from build123d import *

# Parameters (mm, degrees)
CYLINDER004_R     = 28
CYLINDER004_DEPTH = 10


with BuildPart() as cylinder004:
    # Cylinder004 → Cylinder004 (new body)
    with BuildSketch(Plane.XY.offset(86)):
        Circle(CYLINDER004_R)
    extrude(amount=CYLINDER004_DEPTH)


with BuildPart() as cut004:
    # Cone004 → Cone004 (revolve)
    with BuildSketch(Plane(origin=(0, 0, 87), x_dir=(1, 0, 0), z_dir=(0, -1, 0))):
        Polygon((0, 0), (32.6, 0), (33, 5), (0, 5), align=None)
    revolve(axis=Axis((0, 0, 87), (0, 0, 1)))

    # Cut004: cut Cylinder004
    add(cylinder004.part, mode=Mode.SUBTRACT)


solid = cut004.part
Read the model definition and answer for the solid it produces. Units are mm, in the model's axes. Coordinates: 2 decimals unless noted, no trailing zeros. Order: outer loops, then holes, each group sorted by start corner. A loop starts at its lowest first (then second) coordinate and runs counter-clockwise, first axis right, second up. Notation, with made-up numbers: (63.5, -6) -> (100.5, -6) arc R15 cw to (100.5, 23) -> close; hole circle Ø5 at (-2.5, 9.25). An arc over 180 degrees is marked (long way). Answer as a JSON object with one key per item and string values.
1) Each of these flat-tipped pins is pushed along its axis until it touches: pin 1 (12 mm diameter, centred on x = 3.5, y = -18, fed in from +Z); pin 2 (2 mm diameter, centred on y = -14.5, z = 89, fed in from -X). Where does it stop, or does it pass through?
Model answer:
{"pin 1": "passes through", "pin 2": "stops at x = -29.86"}
2) A cutting plane is placed at A-A, the plane y = 0. Determine the outline of the cut face in (x, z), plus the area to 3 significant figures.
Model answer:
{"outline": "(-33, 92) -> (-32.6, 87) -> (-28, 87) -> (-28, 92) -> close; (28, 87) -> (32.6, 87) -> (33, 92) -> (28, 92) -> close", "area": "48.0 mm²"}
3) A cutting plane is placed at C-C, the plane z = 90.6. Determine the outline of the cut face in (x, y).
Model answer:
{"outline": "circle Ø65.78 at (0, 0); hole circle Ø56 at (0, 0)"}
4) The mould has two halves that part along X. Classify faces 1 (the face through (-14.3, 24.3, 87)), 2 (the face through (25.865, -10.724, 89.465)), 3 (the face through (-7.07, -31.85, 87.31)): released by +X, released by -X, zero draft, split by the parting line, or undercut.
Model answer:
{"face 1": "zero draft", "face 2": "undercut", "face 3": "split by the parting line"}
5) Consider line 1 along X through (y, z) = (15.5, 88.7); line 2 along Y through (x, z) = (-8, 88.95); line 3 along X through (y, z) = (22, 89.05). Determine where each line is inside the solid, lowest interval first. Write a range as from..to.
Model answer:
{"line 1": "x = -28.83..-23.32, 23.32..28.83", "line 2": "y = -31.76..-26.83, 26.83..31.76", "line 3": "x = -24.28..-17.32, 17.32..24.28"}
